Geometry check sheet. Reference: drawing and pictorial views, mm from the part's lowest x, y, z. A direction names the side the tool comes from. Coordinates: 2 decimals unless noted, no trailing zeros. Write each loop counter-clockwise with the first axis right and the second up, starting at its lowest first coordinate (ties: lowest second). Pieces come first, ordered by that corner, then holes.
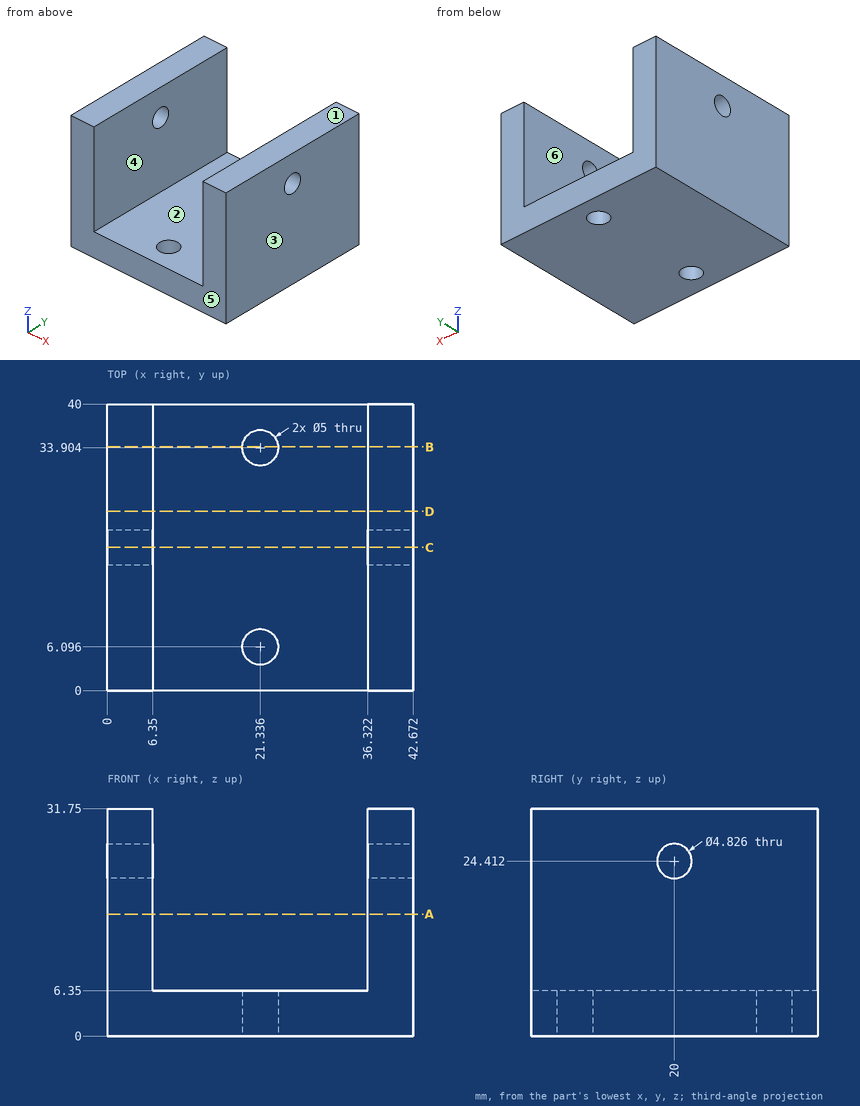
1. Gauge pin test, flat end, axial feed: P1, Ø9, axis at x = 24, y = 14.5, coming from the +Z side. Record the tip position at first contact, or that the pin passes through.
2. Sectioned sample at D-D, the plane y = 25. Record the boundary of the cut face in (x, z).
3. Draft check along X on the marked faces 1, 2, 3 and 4. Enter one of: pulls with the +X half, pulls with the -X half, needs draft (parallel to the pull), parting line crosses it, or undercut.
4. Tool access check on the marked faces 5 and 6. Record the directions out of +Z, -Z, +X, -X, +Y, -Y that give a thin tool (end or side, any length) a straight path to the whole face; none if there is none.
5. Material ranges on L1, parallel to X at y = 36.5, z = 27; L2, parallel to Z at x = 21.5, y = 13.5; L3, parallel to X at y = 8, z = 5.5, recorded low to high.
6. Sectioned sample at C-C, the plane y = 20. Record the boundary of the cut face in (x, z) (3 decimals).
7. Sectioned sample at A-A, the plane z = 17. Record the boundary of the cut face in (x, y).
8. Sectioned sample at B-B, the plane y = 34. Record the boundary of the cut face in (x, z).
Outcome:
1. P1: stops at z = 6.35
2. outline: (0, 0) - (42.67, 0) - (42.67, 31.75) - (36.32, 31.75) - (36.32, 6.35) - (6.35, 6.35) - (6.35, 31.75) - (0, 31.75) - close
3. face 1: needs draft
3. face 2: undercut
3. face 3: pulls with the +X half
3. face 4: undercut
4. face 5: +Z, -Z, +X, -X, -Y
4. face 6: +Z, +Y, -Y
5. L1: x = 0 to 6.35, 36.32 to 42.67
5. L2: z = 0 to 6.35
5. L3: x = 0 to 19.72, 22.96 to 42.67
6. outline: (0, 0) - (42.672, 0) - (42.672, 21.999) - (36.322, 21.999) - (36.322, 6.35) - (6.35, 6.35) - (6.35, 21.999) - (0, 21.999) - close; (0, 26.825) - (6.35, 26.825) - (6.35, 31.75) - (0, 31.75) - close; (36.322, 26.825) - (42.672, 26.825) - (42.672, 31.75) - (36.322, 31.75) - close
7. outline: (0, 0) - (6.35, 0) - (6.35, 40) - (0, 40) - close; (36.32, 0) - (42.67, 0) - (42.67, 40) - (36.32, 40) - close
8. outline: (0, 0) - (18.84, 0) - (18.84, 6.35) - (6.35, 6.35) - (6.35, 31.75) - (0, 31.75) - close; (23.83, 0) - (42.67, 0) - (42.67, 31.75) - (36.32, 31.75) - (36.32, 6.35) - (23.83, 6.35) - close
